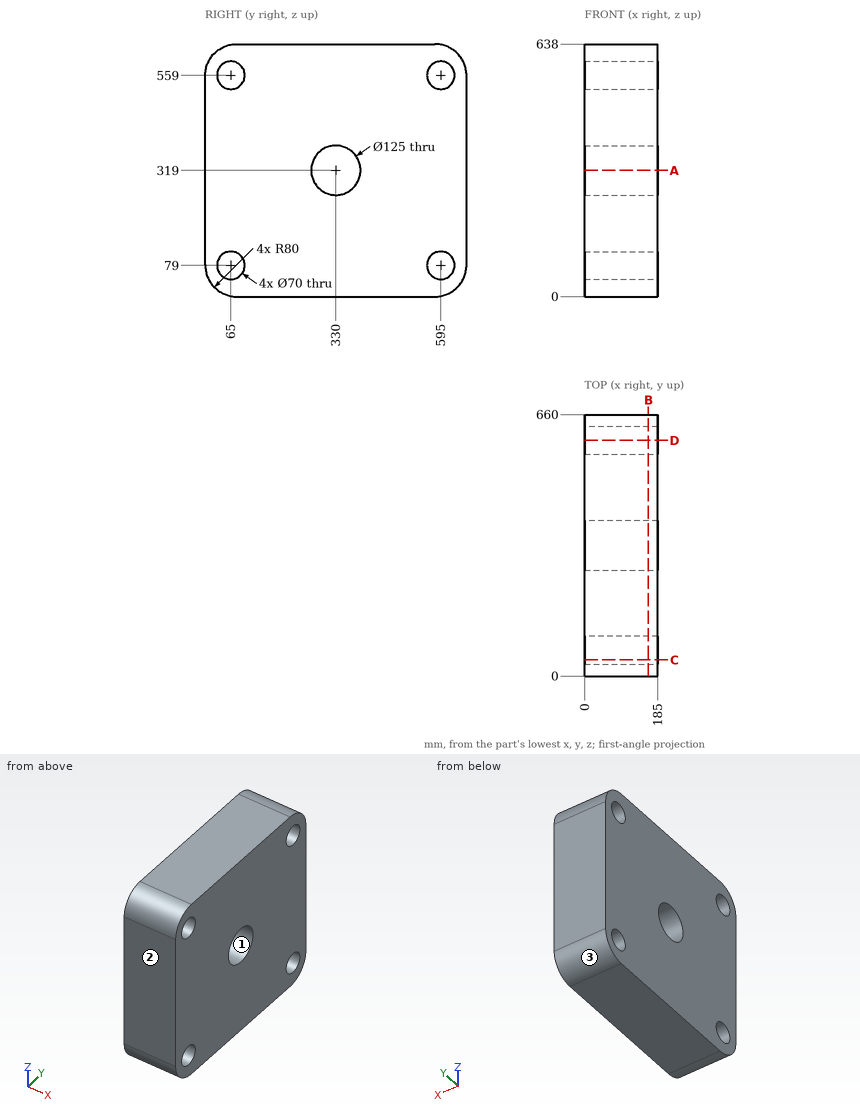
Answer from the drawing. Dimensions are ordinates in mm from the lowest x, y and z of the part. Give positions to 0.01 mm unless a question says otherwise; leave off trailing zeros. Loops run counter-clockwise (first coordinate to the right, second up) from the corner with the lowest first, then second, coordinate; pieces in that order, holes last.
Item 1: The part is cut by section C-C (y = 40.5). Write down the section's boundary in (x, z) (3 decimals), and give its area (3 significant figures).
Item 2: The mould has two halves that part along Y. Classify the marked faces 1, 2 and 3: released by +Y, released by -Y, zero draft, split by the parting line, or undercut.
Item 3: The part is cut by section B-B (x = 161). Write down the section's boundary in (y, z), and give its area (3 significant figures).
Item 4: The part is cut by section D-D (y = 595). Write down the section's boundary in (x, z).
Item 5: Find the intervals of material crossed by line 1 along Z through (x, y) = (48.5, 595); line 2 along Z through (x, y) = (71, 330); line 3 along Y through (x, z) = (51, 351), in increasing order.
Item 6: The part is cut by section A-A (z = 319). Write down the section's boundary in (x, y), and give its area (3 significant figures).
Item 7: This flat-tipped pin is pushed along its axis until it touches: pin 1 Ø4 at (x, y) = (105.5, 70.5) entering from -Z. Where does it stop, or does it pass through?
Taken from the geometry:
1. outline: (0, 10.432) - (185, 10.432) - (185, 54.005) - (0, 54.005) - close; (0, 103.995) - (185, 103.995) - (185, 534.005) - (0, 534.005) - close; (0, 583.995) - (185, 583.995) - (185, 627.568) - (0, 627.568) - close
1. area: 95,700 mm2
2. face 1: undercut
2. face 2: released by -Y
2. face 3: released by +Y
3. outline: (0, 80) arc R80 ccw to (80, 0) - (580, 0) arc R80 ccw to (660, 80) - (660, 558) arc R80 ccw to (580, 638) - (80, 638) arc R80 ccw to (0, 558) - close; hole circle Ø70 at (65, 79); hole circle Ø70 at (65, 559); hole circle Ø125 at (330, 319); hole circle Ø70 at (595, 79); hole circle Ø70 at (595, 559)
3. area: 388,000 mm2
4. outline: (0, 1.42) - (185, 1.42) - (185, 44) - (0, 44) - close; (0, 114) - (185, 114) - (185, 524) - (0, 524) - close; (0, 594) - (185, 594) - (185, 636.58) - (0, 636.58) - close
5. line 1: z = 1.42 to 44, 114 to 524, 594 to 636.58
5. line 2: z = 0 to 256.5, 381.5 to 638
5. line 3: y = 0 to 276.31, 383.69 to 660
6. outline: (0, 0) - (185, 0) - (185, 267.5) - (0, 267.5) - close; (0, 392.5) - (185, 392.5) - (185, 660) - (0, 660) - close
6. area: 99,000 mm2
7. pin 1: stops at z = 0.35
